Geometry check sheet. Reference: the model listing, model coordinates, mm. A direction names the side the tool comes from. Coordinates: 2 decimals unless noted, no trailing zeros. Loops run counter-clockwise (first coordinate to the right, second up) from the corner with the lowest first, then second, coordinate; pieces in that order, holes last. Notation, with made-up numbers: (-23.5, 40.25) - (-0.5, 40.25) arc R19 cw to (-0.5, 46.25) - close; hole circle Ø2 at (86, 20). An arc over 180 degrees is marked (long way). One line per item, written item: value.
Autodesk Inventor part; units mm, degrees
ref_plane "YZ Plane" through (0, 0, 0) normal (1, 0, 0) x (0, 1, 0)
ref_plane "XZ Plane" through (0, 0, 0) normal (0, 1, 0) x (-1, 0, 0)
ref_plane "XY Plane" through (0, 0, 0) normal (0, 0, 1) x (1, 0, 0)
sketch "Sketch1" plane through (0, 0, 0) normal (1, 0, 0) x (0, 1, 0)
  line L0 (-22.9273, 0) -> (27.8727, 0)
  line L1 (27.8727, 0) -> (27.8727, 25.4)
  line L2 (27.8727, 25.4) -> (-22.9273, 25.4)
  line L3 (-22.9273, 25.4) -> (-22.9273, 0)
  line L4 (26.2217, 23.749) -> (-21.2763, 23.749)
  line L5 (-21.2763, 23.749) -> (-21.2763, 1.651)
  line L6 (-21.2763, 1.651) -> (26.2217, 1.651)
  line L7 (26.2217, 1.651) -> (26.2217, 23.749)
  point P0 (0, 0)
  dimension "d0" = 25.4
  dimension "d1" = 50.8
  dimension "d2" = 1.651
  dimension "d3" = 1.651
  dimension "d4" = 1.651
  dimension "d5" = 1.651
extrude "Extrusion1" add sketch "Sketch1" along normal blind 152.4
sketch "Sketch2" plane through (0, -22.9273, 0) normal (0, 0, -1) x (-1, 0, 0)
  circle A0 centre (-63.5, 12.7) radius 2.5797
  circle A1 centre (-88.9, 12.7) radius 2.5797
  circle A2 centre (-38.1, 12.7) radius 2.5797
  circle A3 centre (-12.7, 12.7) radius 2.5797
  circle A4 centre (-114.3, 12.7) radius 2.5797
  circle A5 centre (-139.7, 12.7) radius 2.5797
  line L0 (0, 0) -> (0, 50.8)
  line L1 (-152.4, 0) -> (-152.4, 50.8)
  line L2 (0, 0) -> (-152.4, 0)
  point P0 (0, 22.9273)
  dimension "d8" = 5.1594
  dimension "d9" = 5.1594
  dimension "d13" = 5.1594
  dimension "d14" = 5.1594
  dimension "d15" = 5.1594
  dimension "d16" = 5.1594
  dimension "d17" = 25.4
  dimension "d18" = 12.7
  dimension "d20" = 88.9
  dimension "d21" = 12.7
  dimension "d22" = 12.7
  dimension "d23" = 63.5
  dimension "d24" = 25.4
  dimension "d25" = 12.7
  dimension "d26" = 12.7
  dimension "d27" = 12.7
  dimension "d28" = 12.7
  dimension "d29" = 12.7
extrude "Extrusion2" cut sketch "Sketch2" against normal blind 25.4
equation "\"d3\" = d2"
equation "\"d4\" = d2"
equation "\"d5\" = d2"
equation "\"d9\" = d8"
equation "\"d13\" = d8"
equation "\"d14\" = d8"
equation "\"d15\" = d8"
equation "\"d16\" = d8"
equation "\"d22\" = d21"
equation "\"d26\" = d21"
equation "\"d27\" = d21"
equation "\"d28\" = d21"
equation "\"d29\" = d21"
properties part number "Mounting part"
(1) Release check for a two-part mould opening along Z. For faces 3 (the face through (75, 2, 1.651)), 4 (the face through (137.32, -11.22, 24.56)) record: pulls with the +Z half, pulls with the -Z half, needs draft (parallel to the pull), parting line crosses it, or undercut.
Reply:
face 3: undercut
face 4: needs draft
(2) Cross-section at A-A on x = 12.7. Record the cut outline in (y, z), and give its area (3 significant figures).
Reply:
outline: (-22.93, 0) - (-12.81, 0) - (-12.81, 1.65) - (-21.28, 1.65) - (-21.28, 23.75) - (-12.81, 23.75) - (-12.81, 25.4) - (-22.93, 25.4) - close; (-7.65, 0) - (27.87, 0) - (27.87, 25.4) - (-7.65, 25.4) - (-7.65, 23.75) - (26.22, 23.75) - (26.22, 1.65) - (-7.65, 1.65) - close
area: 224 mm2
(3) Cross-section at D-D on x = 110. Record the cut outline in (y, z).
Reply:
outline: (-22.93, 0) - (27.87, 0) - (27.87, 25.4) - (-22.93, 25.4) - close; hole (-21.28, 1.65) - (26.22, 1.65) - (26.22, 23.75) - (-21.28, 23.75) - close
(4) Material ranges on probe 1 along Y at (x, z) = (67, 23.5); probe 2 along Y at (x, z) = (88.9, 0.85); probe 3 along Z at (x, y) = (109.5, 20), recorded low to high. Write a range as from..to.
Reply:
probe 1: -22.93..-21.28, 26.22..27.87
probe 2: -22.93..-12.81, -7.65..27.87
probe 3: 0..1.65, 23.75..25.4
(5) Cross-section at C-C on z = 16.5. Record the cut outline in (x, y), and give its area (3 significant figures).
Reply:
outline: (0, -22.93) - (152.4, -22.93) - (152.4, -21.28) - (0, -21.28) - close; (0, 26.22) - (152.4, 26.22) - (152.4, 27.87) - (0, 27.87) - close
area: 503 mm2
(6) Access from +Z, -Z, +X, -X, +Y, -Y to the whole of each face (thin tool, end or side, straight path). Record for faces 1 (the face through (75, -22.927, 13)), 2 (the face through (75, -21.276, 13)).
Reply:
face 1: +Z, -Z, +X, -X, -Y
face 2: +X, -X
(7) Cross-section at B-B on y = 5. Record the cut outline in (x, z).
Reply:
outline: (0, 0) - (152.4, 0) - (152.4, 1.65) - (0, 1.65) - close; (0, 23.75) - (152.4, 23.75) - (152.4, 25.4) - (0, 25.4) - close
